Autodesk Inventor part; units mm, degrees
ref_plane "Work Plane1" through (16, 0, 0) normal (1, 0, 0) x (0, 1, 0)
ref_plane "XZ Plane" through (0, 0, 0) normal (0, 1, 0) x (-1, 0, 0)
ref_plane "XY Plane" through (0, 0, 0) normal (0, 0, 1) x (1, 0, 0)
sketch "Sketch1" plane through (0, 0, 0) normal (0, 1, 0) x (-1, 0, 0)
  circle A0 centre (0, 0) radius 16
  dimension "d0" = 32
extrude "Extrusion1" add sketch "Sketch1" along normal blind 70
chamfer "Chamfer1" distance 6 angle 45 1 edges at (16, 70, 0)
chamfer "Chamfer2" distance 11 angle 45 1 edges at (16, 0, 0)
sketch "Sketch2" plane through (0, 70, 0) normal (0, 1, 0) x (1, 0, 0)
  circle A0 centre (0, 0) radius 16
extrude "Extrusion2" add sketch "Sketch2" along normal blind 5
sketch "Sketch3" plane through (0, 0, 0) normal (0, -1, 0) x (1, 0, 0)
  circle A0 centre (0, 0) radius 16
extrude "Extrusion3" add sketch "Sketch3" along normal blind 5
sketch "Sketch4" plane through (0, -5, 0) normal (0, -1, 0) x (1, 0, 0)
  circle A0 centre (0, 0) radius 5
extrude "Extrusion4" add sketch "Sketch4" along normal blind 10
sketch "Sketch5" plane through (0, 75, 0) normal (0, 1, 0) x (1, 0, 0)
  circle A0 centre (0, 0) radius 10
extrude "Extrusion5" add sketch "Sketch5" along normal blind 10
ref_plane "Work Plane1" through (16, 0, 0) normal (1, 0, 0) x (0, 1, 0)
sketch "Sketch6" plane through (16, 0, 0) normal (1, 0, 0) x (0, 1, 0)
  line L0 (11, 16) -> (11, -16)
  line L1 (11, 0) -> (21, 0)
  line L2 (21, 0) -> (21, 7)
  line L3 (11, 16) -> (64, 16)
  line L4 (21, 7) -> (54, 7)
  line L5 (54, 7) -> (54, 16)
  line L6 (54, 16) -> (21, 16)
  line L7 (21, 16) -> (21, 7)
  point P0 (0, 0)
  dimension "d17" = 10
  dimension "d18" = 7
  dimension "d19" = 33
extrude "Extrusion6" cut sketch "Sketch6" against normal through all contours L3 L5 L4 L7
sketch "Sketch7" plane through (-14.3875, 21, 7) normal (0, 0, 1) x (1, 0, 0)
  line L0 (28.775, 0) -> (0, 0)
  line L1 (14.3875, 0) -> (14.3875, 16.5)
  point P0 (14.3875, -21)
  dimension "d22" = 16.5
hole "Hole1" at (0, 37.5, 7) direction (0, 0, -1) diameter 3.242 end through all
properties part number "MMAE 232 Assignment 1e-Nicholas Skiba" material "Aluminum 6061"
The listing builds one solid part. Answer for the finished solid, in the listing's coordinates (mm). A direction names the side the tool comes from. Coordinates: 2 decimals unless noted, no trailing zeros. Order: outer loops, then holes, each group sorted by start corner. A loop starts at its lowest first (then second) coordinate and runs counter-clockwise, first axis right, second up. Notation, with made-up numbers: (88, 44.25) -> (126, 44.25) arc R21 cw to (126, 61.25) -> close; hole circle Ø11 at (-18.5, 59). An arc over 180 degrees is marked (long way). Answer in a Markdown table with one row per item. Add a question column.
Item 1: Find the intervals of material crossed by L1, parallel to Y at x = 0, z = -6.5; L2, parallel to Y at x = 6, z = -13.5; L3, parallel to Y at x = 6, z = 8.5, in increasing order. Write a range as from..to.
Item 2: Find section C-C (y = 37.5). Write down the section's boundary in (x, z), then the cut area to 3 significant figures.
Item 3: Find section B-B (z = 0). Write down the section's boundary in (x, y).
Item 4: Which of the six approach directions +Z, -Z, +X, -X, +Y, -Y give full straight-line access (tool end or side, diameter ignored) to faces 4 (the face through (-1.08, -9.93, 4.88)), 5 (the face through (-0.2, 70, 10.4)), 6 (the face through (-3, 37, 7))?
Item 5: Each of these flat-tipped pins is pushed along its axis until it touches: P1, Ø1.5, axis at y = 45.5, z = 5.5, coming from the -X side; P2, Ø1.5, axis at y = 31.5, z = 9.5, coming from the +X side; P3, Ø4.5, axis at x = -6, z = 11, coming from the -Y side; P4, Ø2, axis at y = 17.5, z = -3.5, coming from the +X side. Where does it stop, or does it pass through?
Item 6: Determine the mould class of faces 1 (the face through (-2.17, 79.93, -9.76)), 2 (the face through (0, 21, 11)), 3 (the face through (-4, -5, 4)) for opening direction Y: +Y half, -Y half, draft (parallel to the pull), parting line (faces both ways), or undercut.
Item 7: Find section D-D (z = -8.5). State how many separate pieces and enclosed holes the cut face has, then the cut area to 3 significant figures.
Result set:
| question | item | result |
|---|---|---|
| 1 | L1 | y = -5..0, 1.5..35.88, 39.12..85 |
| 1 | L2 | y = -5..0, 9.77..65.23, 70..75 |
| 1 | L3 | y = -5..0, 5.4..21, 54..69.6, 70..75 |
| 2 | outline | (-14.39, 7) arc R16 ccw to (-1.62, -15.92) -> (-1.62, 7) -> close; (1.62, -15.92) arc R16 ccw to (14.39, 7) -> (1.62, 7) -> close |
| 2 | area | 544 mm² |
| 3 | outline | (-16, -5) -> (-5, -5) -> (-5, -15) -> (5, -15) -> (5, -5) -> (16, -5) -> (16, 0) -> (5, 0) -> (16, 11) -> (16, 64) -> (10, 70) -> (16, 70) -> (16, 75) -> (10, 75) -> (10, 85) -> (-10, 85) -> (-10, 75) -> (-16, 75) -> (-16, 70) -> (-10, 70) -> (-16, 64) -> (-16, 11) -> (-5, 0) -> (-16, 0) -> close; hole circle Ø3.24 at (0, 37.5) |
| 4 | face 4 | -Y |
| 4 | face 5 | none |
| 4 | face 6 | +Z, +X, -X |
| 5 | P1 | stops at x = -15.28 |
| 5 | P2 | passes through |
| 5 | P3 | stops at y = -5 |
| 5 | P4 | stops at x = 15.8 |
| 6 | face 1 | draft |
| 6 | face 2 | undercut |
| 6 | face 3 | -Y half |
| 7 | separate pieces | 2 |
| 7 | enclosed holes | 1 |
| 7 | area | 2,050 mm² |
